Build history of the part. All positions in model axes, mm. Face numbers are marked on the shaded views. A direction names the side the tool comes from. Round coordinates to 2 decimals unless told otherwise and drop trailing zeros. Order: outer loops, then holes, each group sorted by start corner. A loop starts at its lowest first (then second) coordinate and runs counter-clockwise, first axis right, second up. Notation, with made-up numbers: M -29,74 L -24,74 A11 cw -24,85 Z; hole C 85.5,16 d9. An arc over 180 degrees is marked long. Use CSV: the item, a comma, the result in double quotes.
from build123d import *

# Parameters (mm, degrees)
F0_W     = 7.400000114
F0_H     = 4.400000114
F0_W_2   = 5
F0_H_2   = 2
F1_DEPTH = 0.8
F2_DEPTH = 0.5
F4_R     = 0.2
F5_W     = 0.4
F5_H     = 0.8
F6_DEPTH = 2


# Not quite as in the source:
# - a feature names something its author has since deleted; it is built from what else it names


with BuildPart() as f1:
    # F0 (on Top) → F1 (new body)
    with BuildSketch(Plane.XY):
        with Locations((-2.5, -1)):
            Rectangle(F0_W, F0_H)
        with Locations((-2.5, -1)):
            Rectangle(F0_W_2, F0_H_2, mode=Mode.SUBTRACT)
    extrude(amount=F1_DEPTH)

    # F0 (on Top) → F2 (join)
    with BuildSketch(Plane.XY):
        with Locations((-2.5, -1)):
            Rectangle(F0_W, F0_H)
        with Locations((-2.5, -1)):
            Rectangle(F0_W_2, F0_H_2, mode=Mode.SUBTRACT)
        with Locations((-2.5, -1)):
            Rectangle(F0_W_2, F0_H_2)
    extrude(amount=-F2_DEPTH)

    # F4
    f4_edges = [f1.edges().sort_by_distance(p)[0] for p in [
        (-5, 0, 0.4),
        (0, 0, 0.4),
        (0, -2, 0.4),
        (-5, -2, 0.4),
        (-6.2, 1.2, 0.15),
        (1.2, 1.2, 0.15),
        (1.2, -3.2, 0.15),
        (-6.2, -3.2, 0.15),
    ]]
    fillet(f4_edges, radius=F4_R)

    # F5 (on face) → F6 (join, through all)
    with BuildSketch(Plane.XZ):
        with Locations((-3.6, 0.4)):
            Rectangle(F5_W, F5_H)
    extrude(amount=F6_DEPTH)


solid = f1.part
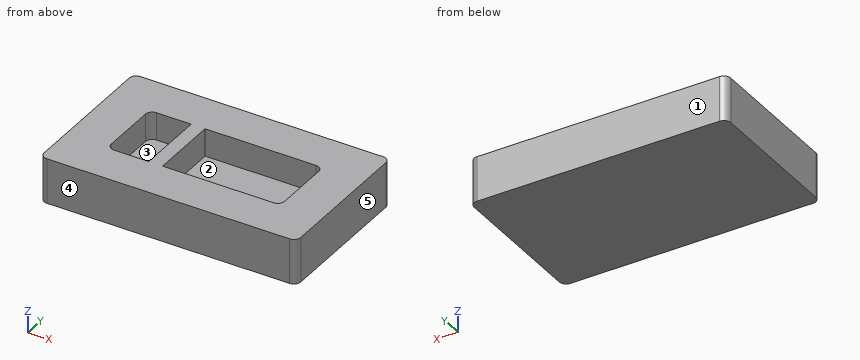
(1) Wall check: line 1 (X direction, y = -0.75, z = 0.05); line 2 (Y direction, x = -0.5, z = 0.3); line 3 (Z direction, x = -1.75, y = -0.3). Give the ranges that are in metal, low to high. Write a range as from..to.
Answer block:
line 1,"x = -6.2..-5, -3.8..-3.4, 0..1.2"
line 2,"y = -3.2..-2, 0..1.2"
line 3,"z = -0.5..0"
(2) Two-plate mould, pull along X, no slides. Class the marked faces 3, 4 and 5: released by +X, released by -X, zero draft, split by the parting line, or undercut.
Answer block:
face 3,"undercut"
face 4,"zero draft"
face 5,"released by +X"
(3) Cut at C-C, the plane x = -3.25. Give the cut face in (y, z).
Answer block:
outline,"M -3.2,-0.5 L 1.2,-0.5 L 1.2,0.8 L 0,0.8 L 0,0 L -2,0 L -2,0.8 L -3.2,0.8 Z"
(4) Cut at B-B, the plane y = -1.25. Give the cut face in (x, z).
Answer block:
outline,"M -6.2,-0.5 L 1.2,-0.5 L 1.2,0.8 L 0,0.8 L 0,0 L -3.4,0 L -3.4,0.8 L -3.8,0.8 L -3.8,0 L -5,0 L -5,0.8 L -6.2,0.8 Z"
(5) Tool access for the marked faces 1 and 2: list every direction of +Z, -Z, +X, -X, +Y, -Y with a clear straight run to the whole face (end or side of a thin tool).
Answer block:
face 1,"+Z, -Z, +X, -X, +Y"
face 2,"+Z"
(6) Cut at A-A, the plane z = 0.15. Give the cut face in (x, y), and give its area (3 significant figures).
Answer block:
outline,"M -6.2,-3 A0.2 ccw -6,-3.2 L 1,-3.2 A0.2 ccw 1.2,-3 L 1.2,1 A0.2 ccw 1,1.2 L -6,1.2 A0.2 ccw -6.2,1 Z; hole M -5,-1.8 A0.2 ccw -4.8,-2 L -3.8,-2 L -3.8,0 L -4.8,0 A0.2 ccw -5,-0.2 Z; hole M -3.4,-2 L -0.2,-2 A0.2 ccw 0,-1.8 L 0,-0.2 A0.2 ccw -0.2,0 L -3.4,0 Z"
area,"23.4 mm²"
